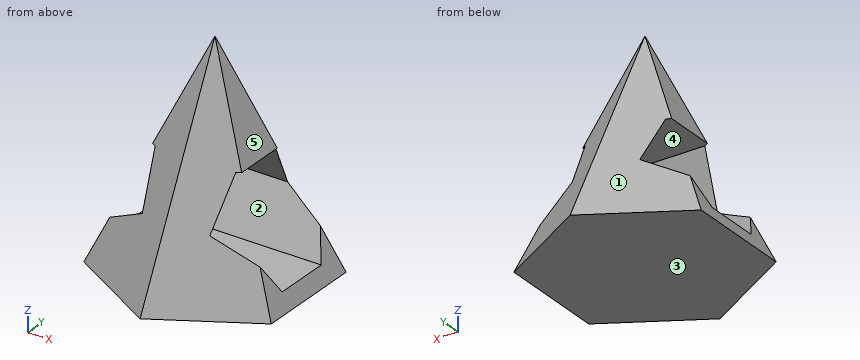
Autodesk Inventor part; units mm, degrees
ref_plane "РабПлоскость1" through (0, 0, 50) normal (0, 0, 1) x (1, 0, 0)
ref_plane "РабПлоскость2" through (25, 0, 0) normal (1, 0, 0) x (0, 1, 0)
ref_plane "XZ Plane" through (0, 0, 0) normal (0, 1, 0) x (-1, 0, 0)
sketch "Эскиз1" plane through (0, 0, 0) normal (0, 0, 1) x (1, 0, 0)
  line L0 (0, -25) -> (-21.6506, -12.5)
  line L1 (-21.6506, -12.5) -> (-21.6506, 12.5)
  line L2 (-21.6506, 12.5) -> (0, 25)
  line L3 (0, 25) -> (21.6506, 12.5)
  line L4 (21.6506, 12.5) -> (21.6506, -12.5)
  line L5 (21.6506, -12.5) -> (0, -25)
  point P0 (0, 0)
  point P1 (0, 0)
ref_plane "РабПлоскость1" through (0, 0, 50) normal (0, 0, 1) x (1, 0, 0)
sketch "Эскиз2" plane through (0, 0, 50) normal (0, 0, 1) x (1, 0, 0)
  point P0 (0, 0)
  point P1 (0, 0)
loft "Лофт1" add profiles "Эскиз1" section 2 point at (0, 0, 50)
ref_plane "РабПлоскость2" through (25, 0, 0) normal (1, 0, 0) x (0, 1, 0)
sketch "Эскиз3" plane through (25, 0, 0) normal (1, 0, 0) x (0, 1, 0)
  line L0 (25, 0) -> (0, 50)
  line L1 (13, 15) -> (6.5, 3.7417)
  line L2 (6.5, 3.7417) -> (-6.5, 3.7417)
  line L3 (-6.5, 3.7417) -> (-13, 15)
  line L4 (-13, 15) -> (-6.5, 26.2583)
  line L5 (-6.5, 26.2583) -> (6.5, 26.2583)
  line L6 (6.5, 26.2583) -> (13, 15)
  point P0 (0, 0)
  point P1 (0, 15)
extrude "Выдавливание1" cut sketch "Эскиз3" against normal blind 50
properties part number "пирамида"
Geometry check sheet. Reference: the model listing, model coordinates, mm. Face numbers are marked on the shaded views. A direction names the side the tool comes from. Give positions to 0.01 mm unless a question says otherwise; leave off trailing zeros. Write each loop counter-clockwise with the first axis right and the second up, starting at its lowest first coordinate (ties: lowest second). Pieces come first, ordered by that corner, then holes. Notation, with made-up numbers: (12.5, -30) -> (59.5, -30) arc R15 cw to (59.5, -8) -> close; hole circle Ø2 at (18.25, -14). An arc over 180 degrees is marked (long way). Use one line per item in the form item = value.
Item 1: Sectioned sample at D-D on z = 43. Enter the section's corners in (x, y).
Results list:
outline = (-3.03, -1.75) -> (0, -3.5) -> (3.03, -1.75) -> (3.03, 1.75) -> (0, 3.5) -> (-3.03, 1.75) -> close
Item 2: Sectioned sample at A-A on z = 22. Enter the section's corners in (x, y).
Results list:
outline = (-8.73, -8.96) -> (0, -14) -> (8.73, -8.96) -> close; (-8.73, 8.96) -> (8.73, 8.96) -> (0, 14) -> close
Item 3: Access from +Z, -Z, +X, -X, +Y, -Y to the whole of each face (thin tool, end or side, straight path). Record for the marked faces 4 and 5.
Results list:
face_4 = +X, -X
face_5 = +Z, +X, +Y, -Y
Item 4: Sectioned sample at B-B on y = 1.5. Enter the section's corners in (x, z).
Results list:
outline = (-21.65, 0) -> (21.65, 0) -> (20.03, 3.74) -> (-20.03, 3.74) -> close; (-10.28, 26.26) -> (10.28, 26.26) -> (2.6, 44) -> (0, 47) -> (-2.6, 44) -> close
Item 5: Sectioned sample at C-C on x = -5. Enter the section's corners in (y, z).
Results list:
outline = (-22.11, 0) -> (22.11, 0) -> (2.89, 38.45) -> (-2.89, 38.45) -> close; hole (-13, 15) -> (-6.5, 3.74) -> (6.5, 3.74) -> (13, 15) -> (6.5, 26.26) -> (-6.5, 26.26) -> close
Item 6: Depth check by flat-ended pin: pin 1 Ø4 at (x, z) = (-12, 12.5) entering from +Y; pin 2 Ø1.5 at (x, z) = (7.5, 8) entering from -Y; pin 3 Ø2 at (x, y) = (7.5, -5) entering from +Z; pin 4 Ø14.5 at (x, y) = (-3.5, 3) entering from -Z. Enter the tip coordinate at first touch or a pass-through.
Results list:
pin_1 = 13.35
pin_2 = -17.24
pin_3 = 33.65
pin_4 = 0
Item 7: Mould release check, pull along Z, two halves, no side actions. Record for the marked faces 1, 2 and 3: released by +Z, released by -Z, zero draft, split by the parting line, or undercut.
Results list:
face_1 = released by +Z
face_2 = undercut
face_3 = released by -Z
Item 8: Scan lines: line 1 (Z direction, x = 5, y = -3); line 2 (Z direction, x = 5.5, y = 10.5); line 3 (Z direction, x = 10.5, y = 4.5). Record each from-to range of solid material in increasing order.
Results list:
line_1 = 0 to 3.74, 26.26 to 38.23
line_2 = 0 to 10.67, 19.33 to 22.65
line_3 = 0 to 3.74
